from build123d import *

# Parameters (mm, degrees)
F0_W          = 38.1
F0_H          = 38.1
F1_DEPTH      = 304.8
F1_DEPTH_BACK = 304.8
F2_W          = 38.1
F2_H          = 4.7625
F3_DEPTH      = 38.101
F5_D          = 7.9375
F7_DEPTH      = 609.601


with BuildPart() as f1:
    # F0 (on Right) → F1 (new body, two sides)
    with BuildSketch(Plane.YZ) as f1_sk:
        with Locations((19.05, 19.05)):
            Rectangle(F0_W, F0_H)
    extrude(amount=F1_DEPTH)
    extrude(f1_sk.sketch, amount=-F1_DEPTH_BACK)

    # F2 (on face) → F3 (cut, through all)
    with BuildSketch(Plane.XY.offset(38.1)):
        with Locations((-50.8, 2.38125)):
            Rectangle(F2_W, F2_H)
        with Locations((276.225, 2.38125)):
            Rectangle(F2_W, F2_H)
    extrude(amount=-F3_DEPTH, mode=Mode.SUBTRACT)

    # F5 (through all)
    with Locations(Plane.XZ.offset(-4.7625)):
        with Locations((-50.8, 19.05), (276.225, 19.05)):
            Hole(F5_D / 2)

    # F6 (on face) → F7 (cut, through all)
    with BuildSketch(Plane.YZ.offset(304.8)):
        Polygon((38.1, 0), (38.1, 38.1), (16.102955, 0), align=None)
    extrude(amount=-F7_DEPTH, mode=Mode.SUBTRACT)


solid = f1.part
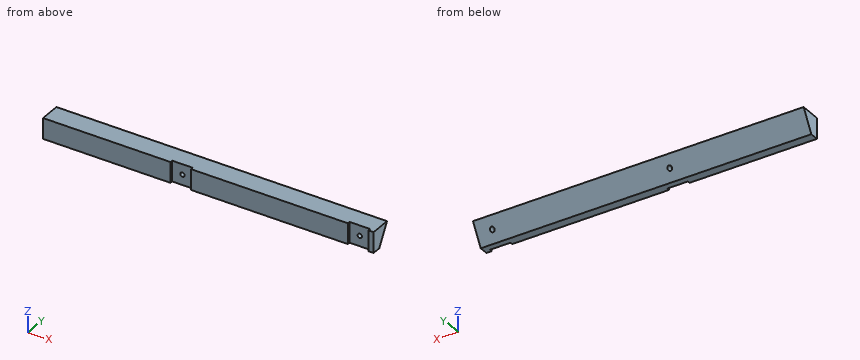
Verification items for the finished model (mm, model axes). Coordinates: 2 decimals unless noted, no trailing zeros. Order: outer loops, then holes, each group sorted by start corner. A loop starts at its lowest first (then second) coordinate and runs counter-clockwise, first axis right, second up. Notation, with made-up numbers: M -27.5,-20 L -2.5,-20 A25 cw -2.5,12 Z; hole C 26,72 d2. An arc over 180 degrees is marked long. One line per item, written item: value. Start each with the question number.
Item 1: Depth check by flat-ended pin: P1, Ø4, axis at x = 195, y = 19, coming from the -Z side. Enter the tip coordinate at first touch or a pass-through.
Item 2: Sectioned sample at B-B on x = 6. Record the cut outline in (y, z).
Item 3: Thickness scan on probe 1 along X at (y, z) = (17.5, 20); probe 2 along X at (y, z) = (18, 19); probe 3 along Z at (x, y) = (-50.8, 14.25). Record the ranges inside material, lowest first.
Calculated:
1. P1: z = 1.55
2. outline: M 0,0 L 16.1,0 L 38.1,38.1 L 0,38.1 Z
3. probe 1: -304.8 to -54.65, -46.95 to 272.37, 280.08 to 304.8
3. probe 2: -304.8 to -54.77, -46.83 to 272.26, 280.19 to 304.8
3. probe 3: 0 to 15.08, 23.02 to 38.1
